from build123d import *

# Parameters (mm, degrees)
SKETCH_6_W          = 440
SKETCH_6_H          = 200
SKETCH_6_R          = 40
EXTRUDE_2_DEPTH     = 6
SKETCH_7_R          = 2.25
CUT_EXTRUDE_1_DEPTH = 10


with BuildPart() as part:
    # 草图6 → 凸台-拉伸2 (new body)
    with BuildSketch(Plane(origin=(0, 0, 0), x_dir=(1, 0, 0), z_dir=(0, 1, 0))):
        Rectangle(SKETCH_6_W, SKETCH_6_H)
        with Locations(Location((0, 0, 0), (0, 0, 270))):
            Circle(SKETCH_6_R, mode=Mode.SUBTRACT)
    extrude(amount=EXTRUDE_2_DEPTH)

    # 草图7 → 切除-拉伸1 (cut)
    with BuildSketch(Plane(origin=(0, 6, 0), x_dir=(1, 0, 0), z_dir=(0, 1, 0))):
        with BuildLine():
            Line((-220, 100), (-220, 50))
            ThreePointArc((-220, 50), (-205.355339059, 85.355339059), (-170, 100))
            Line((-170, 100), (-220, 100))
        make_face()
        with BuildLine():
            ThreePointArc((-170, -100), (-205.355339059, -85.355339059), (-220, -50))
            Line((-220, -50), (-220, -100))
            Line((-220, -100), (-170, -100))
        make_face()
        with BuildLine():
            Line((220, 100), (170, 100))
            ThreePointArc((170, 100), (205.355339059, 85.355339059), (220, 50))
            Line((220, 50), (220, 100))
        make_face()
        with BuildLine():
            ThreePointArc((220, -50), (205.355339059, -85.355339059), (170, -100))
            Line((170, -100), (220, -100))
            Line((220, -100), (220, -50))
        make_face()
        with Locations(Location((170, 35, 0), (0, 0, 270))):
            Circle(SKETCH_7_R)
        with Locations(Location((200, 35, 0), (0, 0, 270))):
            Circle(SKETCH_7_R)
        with Locations(Location((180, 70, 0), (0, 0, 270))):
            Circle(SKETCH_7_R)
        with Locations(Location((-180, 70, 0), (0, 0, 270))):
            Circle(SKETCH_7_R)
        with Locations(Location((-200, 35, 0), (0, 0, 270))):
            Circle(SKETCH_7_R)
        with Locations(Location((-170, 35, 0), (0, 0, 270))):
            Circle(SKETCH_7_R)
        with Locations(Location((-170, -35, 0), (0, 0, 270))):
            Circle(SKETCH_7_R)
        with Locations(Location((-200, -35, 0), (0, 0, 270))):
            Circle(SKETCH_7_R)
        with Locations(Location((-180, -70, 0), (0, 0, 270))):
            Circle(SKETCH_7_R)
        with Locations(Location((180, -70, 0), (0, 0, 270))):
            Circle(SKETCH_7_R)
        with Locations(Location((200, -35, 0), (0, 0, 270))):
            Circle(SKETCH_7_R)
        with Locations(Location((170, -35, 0), (0, 0, 270))):
            Circle(SKETCH_7_R)
    extrude(amount=-CUT_EXTRUDE_1_DEPTH, mode=Mode.SUBTRACT)


solid = part.part
The model under review builds one solid part; all positions refer to its coordinate system, in mm. Round coordinates to 2 decimals unless told otherwise and drop trailing zeros. Loops run counter-clockwise (first coordinate to the right, second up) from the corner with the lowest first, then second, coordinate; pieces in that order, holes last. Notation, with made-up numbers: (59.25, 52.5) - (87.25, 52.5) arc R15 ccw to (87.25, 73.5) - close; hole circle Ø10 at (38.25, 33.25). An arc over 180 degrees is marked (long way). Use CSV: the item, a comma, the result in double quotes.
(1) Take a section at B-B, the plane x = -18.5. Give the boundary of the cut face in (y, z), plus the area to 3 significant figures.
Working result:
outline,"(0, -100) - (6, -100) - (6, -35.46) - (0, -35.46) - close; (0, 35.46) - (6, 35.46) - (6, 100) - (0, 100) - close"
area,"774 mm^2"
(2) Clearance check with flat-ended pins moving along their axes: P1, Ø4, axis at x = -200, z = 35, coming from the +Y side; P2, Ø2, axis at y = 3, z = 51.5, coming from the -X side. State where each tip first meets the part, or that it passes through.
Working result:
P1,"passes through"
P2,"stops at x = -220"
(3) Take a section at A-A, the plane y = 3.95. State how many separate pieces and enclosed holes the cut face has, plus the area to 3 significant figures.
Working result:
separate pieces,"1"
enclosed holes,"13"
area,"80,600 mm^2"
(4) The part is to be moulded in two halves that separate along X. For faces 1 (the flat face through (-3, 0, -46)), 2 (the cylindrical face through (205.742, 3.042, 84.964)), 3 (the cylindrical face through (-39.05, 2.96, -8.67)), say which applies: pulls with the +X half, pulls with the -X half, needs draft (parallel to the pull), parting line crosses it, or undercut.
Working result:
face 1,"needs draft"
face 2,"pulls with the +X half"
face 3,"undercut"
(5) Take a section at C-C, the plane z = -0.5. Give the boundary of the cut face in (x, y).
Working result:
outline,"(-220, 0) - (-40, 0) - (-40, 6) - (-220, 6) - close; (40, 0) - (220, 0) - (220, 6) - (40, 6) - close"
(6) For line 1 (Z direction, x = 1, y = 1.4); line 2 (X direction, y = 1.8, z = -35); line 3 (X direction, y = 3.1, z = -23), list the stretches that pass through material, from the lowest coordinate up.
Working result:
line 1,"z = -100 to -39.99, 39.99 to 100"
line 2,"x = -220 to -202.25, -197.75 to -172.25, -167.75 to -19.36, 19.36 to 167.75, 172.25 to 197.75, 202.25 to 220"
line 3,"x = -220 to -32.73, 32.73 to 220"
